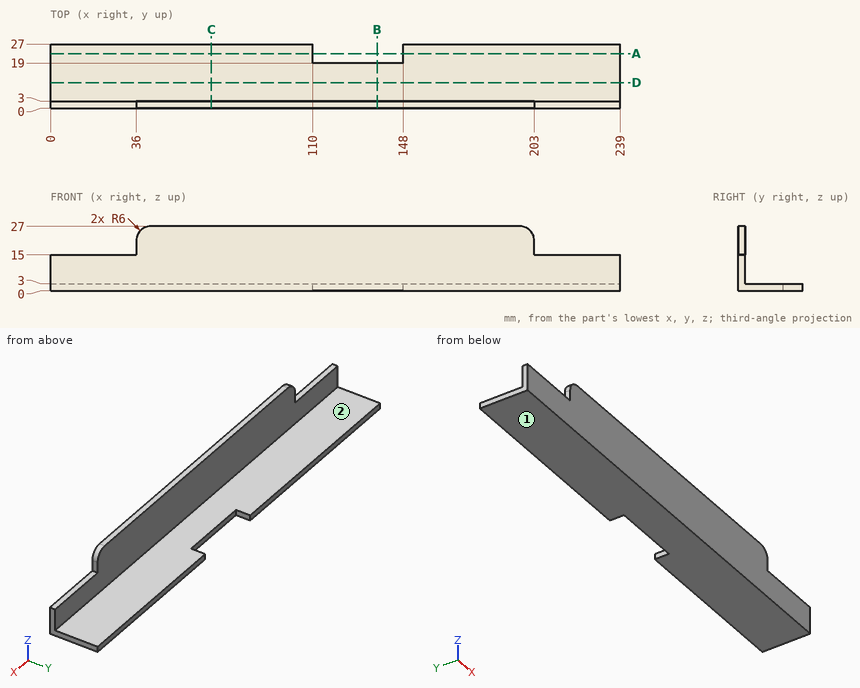
Can you work these out from the drawing? Everything is in mm from the part's minimum corner. A direction names the side the tool comes from. Give positions to 0.01 mm unless a question says otherwise; leave off trailing zeros. Order: outer loops, then holes, each group sorted by start corner. A loop starts at its lowest first (then second) coordinate and runs counter-clockwise, first axis right, second up. Notation, with made-up numbers: M -25.75,53 L 9.25,53 A20 ccw 9.25,58 Z; hole C -9,-3.75 d11. An arc over 180 degrees is marked long. One line per item, written item: value.
Item 1: For pin 1 (0.9 mm diameter, centred on x = 136.5, z = 2, fed in from +Y); pin 2 (2 mm diameter, centred on x = 186, z = 11.5, fed in from +Y); pin 3 (4 mm diameter, centred on x = 111.5, y = 15, fed in from +Z); pin 4 (2 mm diameter, centred on y = 4.5, z = 19.5, fed in from -X), each with a flat end and sliding along its axis, tell me the tip position at first contact or that it passes through.
Verdict:
pin 1: y = 19
pin 2: y = 3
pin 3: z = 3
pin 4: through
Item 2: If we section it at A-A on y = 23: Write out the boundary of the cut face in (x, z).
Verdict:
outline: M 0,0 L 110,0 L 110,3 L 0,3 Z; M 148,0 L 239,0 L 239,3 L 148,3 Z
Item 3: If we section it at B-B on x = 137: Write out the boundary of the cut face in (y, z).
Verdict:
outline: M 0,0 L 19,0 L 19,3 L 3,3 L 3,27 L 0,27 Z
Item 4: For the marked faces 1 and 2, which set-ups out of +Z, -Z, +X, -X, +Y, -Y let a thin tool reach every point of the face, with its end or its side?
Verdict:
face 1: -Z, +X, -X, +Y, -Y
face 2: +Z, +X, -X, +Y
Item 5: Please list where these lines run through material, in increasing order: line 1 (Z direction, x = 178, y = 4); line 2 (X direction, y = 1.75, z = 21.5).
Verdict:
line 1: 0 to 3
line 2: 36.02 to 202.98
Item 6: If we section it at D-D on y = 10.75: Write out the boundary of the cut face in (x, z).
Verdict:
outline: M 0,0 L 239,0 L 239,3 L 0,3 Z
Item 7: If we section it at C-C on x = 67.5: Write out the boundary of the cut face in (y, z), and give its area (3 significant figures).
Verdict:
outline: M 0,0 L 27,0 L 27,3 L 3,3 L 3,27 L 0,27 Z
area: 153 mm2
